Geometry: final body of the model. Coordinates: model frame, mm. A direction names the side the tool comes from. Give positions to 0.01 mm unless a question says otherwise; leave off trailing zeros. Order: outer loops, then holes, each group sorted by start corner. A loop starts at its lowest first (then second) coordinate and runs counter-clockwise, first axis right, second up. Notation, with made-up numbers: (52.25, 42) -> (57.25, 42) arc R34 ccw to (57.25, 72) -> close; hole circle Ø4 at (-20, 62.25). An arc over 180 degrees is marked (long way). Write item = value, one per line.
```python
from build123d import *

# Parameters (mm, degrees)
F0_R     = 4.953
F1_DEPTH = 12.7
F4_DEPTH = 44.45


with BuildPart() as f1:
    # F0 (on Front) → F1 (new body)
    with BuildSketch(Plane.XZ):
        with BuildLine():
            ThreePointArc((0, 12.7), (3.719744, 3.719744), (12.7, 0))
            Line((12.7, 0), (50.8, 0))
            ThreePointArc((50.8, 0), (59.780256, 3.719744), (63.5, 12.7))
            Line((63.5, 12.7), (63.5, 32.512))
            Line((63.5, 32.512), (63.5, 45.212))
            Line((63.5, 45.212), (63.5, 76.2))
            ThreePointArc((63.5, 76.2), (59.780256, 85.180256), (50.8, 88.9))
            Line((50.8, 88.9), (12.7, 88.9))
            ThreePointArc((12.7, 88.9), (3.719744, 85.180256), (0, 76.2))
            Line((0, 76.2), (0, 12.7))
        make_face()
        with Locations((12.7, 12.7)):
            Circle(F0_R, mode=Mode.SUBTRACT)
        Polygon((33.909, 71.006829), (56.134, 32.512), (28.637693, 16.637), (6.412693, 55.131829), align=None, mode=Mode.SUBTRACT)
        with Locations((50.8, 12.7)):
            Circle(F0_R, mode=Mode.SUBTRACT)
        with Locations((12.7, 76.2)):
            Circle(F0_R, mode=Mode.SUBTRACT)
        with Locations((50.8, 76.2)):
            Circle(F0_R, mode=Mode.SUBTRACT)
        Polygon((28.637693, 16.637), (56.134, 32.512), (33.909, 71.006829), (6.412693, 55.131829), align=None)
    extrude(amount=-F1_DEPTH)

    # F3 (on face) → F4 (join, through all)
    with BuildSketch(Plane(origin=(-0.044609, 0, 0.077265), x_dir=(0.866025, 0, 0.5), z_dir=(-0.5, 0, 0.866025))):
        Polygon((64.86947, 0), (33.11947, 0), (33.11947, -14.732), (33.11947, -33.782), (36.42147, -33.782), (45.81947, -21.082), (45.81947, -14.732), (48.99447, -14.732), (52.16947, -14.732), (52.16947, -21.082), (61.56747, -33.782), (64.86947, -33.782), align=None)
    extrude(amount=F4_DEPTH)


solid = f1.part
```
1) Mould query, pull axis X, two halves, no side actions, for faces 5 (the face through (19, -33.782, 36)), 6 (the face through (50.16, 6.26, 81.11)), 7 (the face through (3.82, 6.26, 85.28)), 8 (the face through (34.2, -17.9, 45.1)). Classes: +X half, -X half, draft (parallel to the pull), parting line (faces both ways), or undercut.
Check sheet entries:
face_5 = draft
face_6 = undercut
face_7 = -X half
face_8 = undercut
2) Reachability of faces 1 (the face through (17.681, -16.655, 35.615)), 2 (the face through (24.553, -27.521, 39.583)), 3 (the face through (3.62, 6.26, 3.82)), 4 (the face through (42.19, -12.9, 24.46)) from +Z, -Z, +X, -X, +Y, -Y: full face, straight path, thin tool, end or side. Return the list, or none.
Check sheet entries:
face_1 = -Z, -X, -Y
face_2 = -Y
face_3 = -Z, -X, +Y, -Y
face_4 = -Z, +X, -Y
3) First-contact query: P1, Ø9, axis at x = 12.7, z = 76.2, coming from the +Y side; P2, Ø13, axis at x = 12.7, z = 12.7, coming from the -Y side; P3, Ø5, axis at y = -15.5, z = 62.5, coming from the -X side. Flat tips, straight axial feed; report the tip coordinate or a pass-through.
Check sheet entries:
P1 = through
P2 = 0
P3 = 14.84
4) Line query: line 1 (Z direction, x = 12.7, y = 7); line 2 (Z direction, x = 50, y = 8); line 3 (X direction, y = 10, z = 12). Output: solid intervals per line, ascending. Write a range as from..to.
Check sheet entries:
line_1 = 0..7.75, 17.65..71.25, 81.15..88.9
line_2 = 0..7.81, 17.59..71.31, 81.09..88.9
line_3 = 0.02..7.8, 17.6..45.9, 55.7..63.48
5) Section query C-C (x = 20). Output: boundary loops of the cut face in (y, z).
Check sheet entries:
outline = (-33.78, 31.6) -> (0, 31.6) -> (0, 0) -> (12.7, 0) -> (12.7, 88.9) -> (0, 88.9) -> (0, 62.98) -> (-14.73, 62.98) -> (-14.73, 57) -> (-21.08, 57) -> (-33.78, 38.2) -> close
6) Section query B-B (y = 7). Output: boundary loops of the cut face in (x, z).
Check sheet entries:
outline = (0, 12.7) arc R12.7 ccw to (12.7, 0) -> (50.8, 0) arc R12.7 ccw to (63.5, 12.7) -> (63.5, 76.2) arc R12.7 ccw to (50.8, 88.9) -> (12.7, 88.9) arc R12.7 ccw to (0, 76.2) -> close; hole circle Ø9.91 at (12.7, 12.7); hole circle Ø9.91 at (12.7, 76.2); hole circle Ø9.91 at (50.8, 12.7); hole circle Ø9.91 at (50.8, 76.2)
7) Section query D-D (z = 48.5). Output: boundary loops of the cut face in (x, y), plus the area to 3 significant figures.
Check sheet entries:
outline = (0, 0) -> (10.24, 0) -> (10.24, -33.78) -> (14.05, -33.78) -> (24.91, -21.08) -> (24.91, -14.73) -> (32.24, -14.73) -> (32.24, -21.08) -> (43.09, -33.78) -> (46.9, -33.78) -> (46.9, 0) -> (63.5, 0) -> (63.5, 12.7) -> (0, 12.7) -> close
area = 1,770 mm²
8) Section query A-A (y = -17). Output: boundary loops of the cut face in (x, z), plus the area to 3 significant figures.
Check sheet entries:
outline = (6.41, 55.13) -> (28.64, 16.64) -> (39.64, 22.99) -> (17.41, 61.48) -> close; (22.91, 64.66) -> (45.14, 26.16) -> (56.13, 32.51) -> (33.91, 71.01) -> close
area = 1,130 mm²
